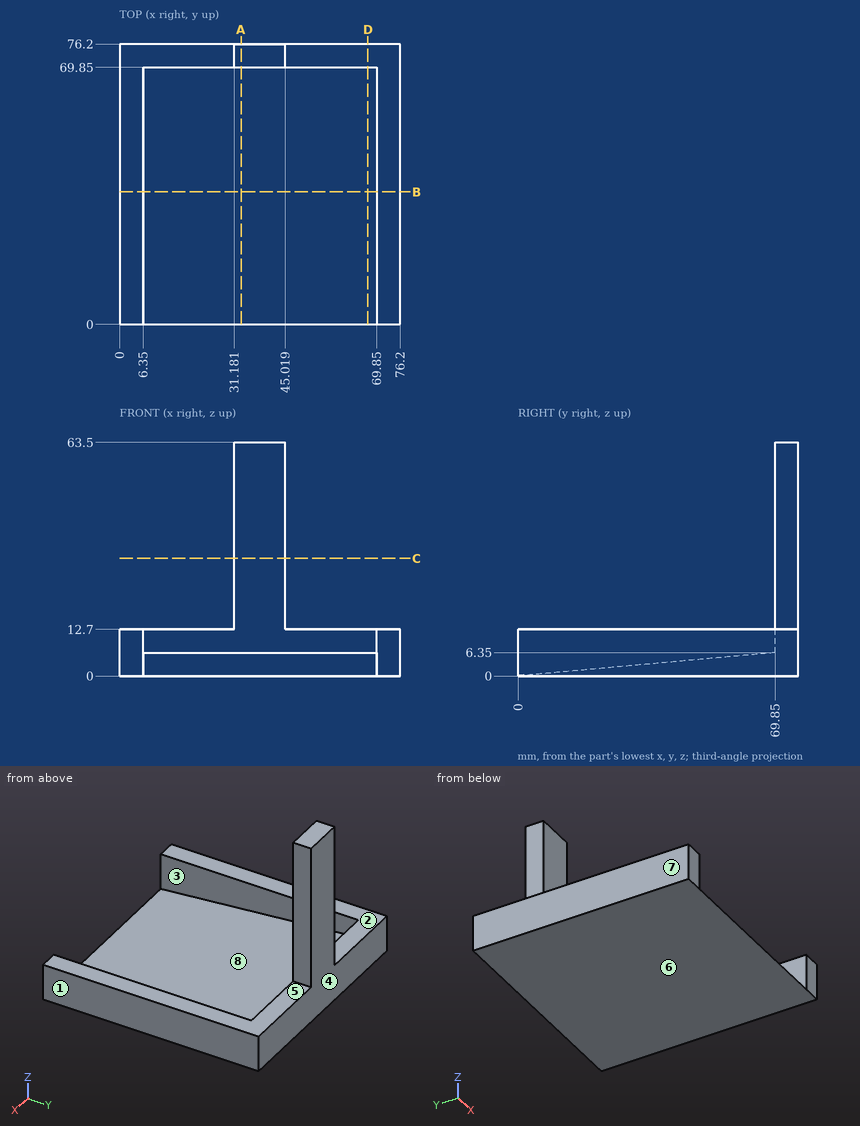
Verification items for this drawing (mm, ordinates from the low corner). A direction names the side the tool comes from. Give positions to 0.01 mm unless a question says otherwise; leave off trailing zeros. Write each loop counter-clockwise with the first axis right and the second up, starting at its lowest first coordinate (ties: lowest second). Pieces come first, ordered by that corner, then holes.
1) Access from +Z, -Z, +X, -X, +Y, -Y to the whole of each face (thin tool, end or side, straight path). Record for the marked faces 1, 2, 3, 4 and 5.
2) Section check C-C, the plane z = 32. Record the boundary of the cut face in (x, y).
3) Section check A-A, the plane x = 33. Record the boundary of the cut face in (y, z).
4) Release check for a two-part mould opening along X. For the marked faces 6, 7 and 8 record: pulls with the +X half, pulls with the -X half, needs draft (parallel to the pull), parting line crosses it, or undercut.
5) Section check D-D, the plane x = 67.5. Record the boundary of the cut face in (y, z).
6) Gauge pin test, flat ends, axial feed: pin 1 (5 mm diameter, centred on y = 72.5, z = 40, fed in from -X); pin 2 (12 mm diameter, centred on x = 19, z = 18, fed in from +Y); pin 3 (1 mm diameter, centred on x = 14, y = 12, fed in from +Z); pin 4 (9.5 mm diameter, centred on x = 10.5, y = 54.5, fed in from +Z). Record the tip position at first contact, or that the pin passes through.
7) Section check B-B, the plane y = 36. Record the boundary of the cut face in (x, z).
8) Material ranges on L1, parallel to X at y = 38, z = 7.5; L2, parallel to Z at x = 70, y = 9; L3, parallel to Y at x = 31.5, z = 47, recorded low to high.
Computed:
1. face 1: +Z, -Z, +X, +Y, -Y
1. face 2: +Z, -X, +Y, -Y
1. face 3: +Z, -Y
1. face 4: +Z, -Z, +X, -X, +Y
1. face 5: +Z, +X, +Y, -Y
2. outline: (31.18, 69.85) - (45.02, 69.85) - (45.02, 76.2) - (31.18, 76.2) - close
3. outline: (0, 0) - (76.2, 0) - (76.2, 63.5) - (69.85, 63.5) - (69.85, 6.35) - close
4. face 6: needs draft
4. face 7: pulls with the -X half
4. face 8: undercut
5. outline: (0, 0) - (76.2, 0) - (76.2, 12.7) - (69.85, 12.7) - (69.85, 6.35) - close
6. pin 1: stops at x = 31.18
6. pin 2: stops at y = 76.2
6. pin 3: stops at z = 1.14
6. pin 4: stops at z = 12.7
7. outline: (0, 0) - (76.2, 0) - (76.2, 12.7) - (69.85, 12.7) - (69.85, 3.27) - (6.35, 3.27) - (6.35, 12.7) - (0, 12.7) - close
8. L1: x = 0 to 6.35, 69.85 to 76.2
8. L2: z = 0 to 12.7
8. L3: y = 69.85 to 76.2
